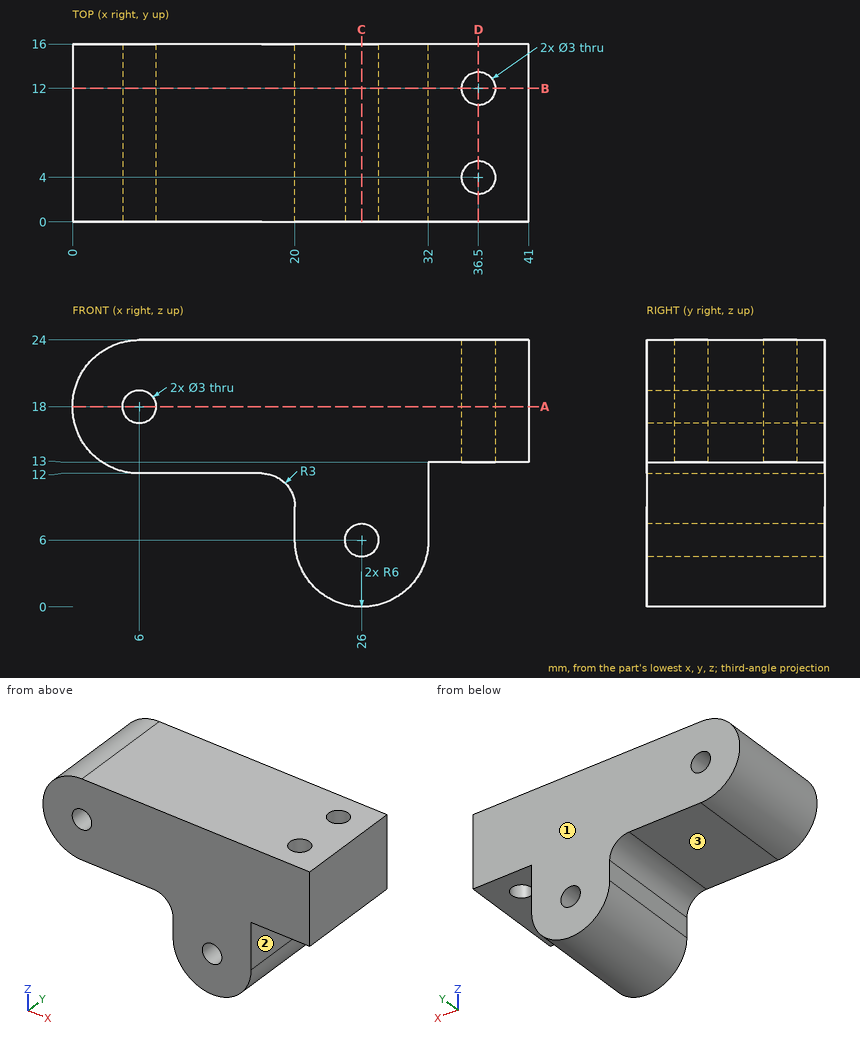
For this review, use the dimensioned drawing (mm, ordinates from the lowest corner) and the shaded views. A direction names the side the tool comes from. Round coordinates to 2 decimals unless told otherwise and drop trailing zeros. Order: outer loops, then holes, each group sorted by start corner. A loop starts at its lowest first (then second) coordinate and runs counter-clockwise, first axis right, second up. Notation, with made-up numbers: (6, -15.75) -> (53, -15.75) arc R29 ccw to (53, 14.25) -> close; hole circle Ø1 at (-20, -38.5). An arc over 180 degrees is marked (long way). One line per item, written item: value. Start each with the question number.
Q1. Take a section at C-C (x = 26). Write out the cut boundary in (y, z).
Q2. Clearance check with flat-ended pins moving along their axes: pin 1 Ø2.5 at (x, z) = (26, 6) entering from -Y; pin 2 Ø5.5 at (y, z) = (6.5, 9.5) entering from +X; pin 3 Ø1.5 at (y, z) = (10.5, 8) entering from -X; pin 4 Ø5.5 at (x, y) = (10, 5.5) entering from -Z. State where each tip first meets the part, or that it passes through.
Q3. Wall thickness on line 1 (Y direction, x = 36.5, z = 20.75); line 2 (X direction, y = 4.75, z = 18); line 3 (X direction, y = 10, z = 6): over which ranges is each line inside the solid? List them lowest first.
Q4. Take a section at D-D (x = 36.5). Write out the cut boundary in (y, z).
Q5. Machinability: for the marked faces 1, 2 and 3, which of the approach directions +Z, -Z, +X, -X, +Y, -Y give a long, thin tool a straight path to every point of the face, cutting with its end or side? Answer none if there is none.
Q6. Take a section at A-A (z = 18). Write out the cut boundary in (x, y), and give its area (3 significant figures).
Q7. Take a section at B-B (y = 12). Write out the cut boundary in (x, z).
Reported:
1. outline: (0, 0) -> (16, 0) -> (16, 4.5) -> (0, 4.5) -> close; (0, 7.5) -> (16, 7.5) -> (16, 24) -> (0, 24) -> close
2. pin 1: passes through
2. pin 2: stops at x = 32
2. pin 3: stops at x = 20
2. pin 4: stops at z = 12
3. line 1: y = 0 to 2.5, 5.5 to 10.5, 13.5 to 16
3. line 2: x = 0 to 4.5, 7.5 to 35.2, 37.8 to 41
3. line 3: x = 20 to 24.5, 27.5 to 32
4. outline: (0, 13) -> (2.5, 13) -> (2.5, 24) -> (0, 24) -> close; (5.5, 13) -> (10.5, 13) -> (10.5, 24) -> (5.5, 24) -> close; (13.5, 13) -> (16, 13) -> (16, 24) -> (13.5, 24) -> close
5. face 1: +Z, -Z, +X, -X, +Y
5. face 2: -Z, +X, +Y, -Y
5. face 3: -Z, -X, +Y, -Y
6. outline: (0, 0) -> (4.5, 0) -> (4.5, 16) -> (0, 16) -> close; (7.5, 0) -> (41, 0) -> (41, 16) -> (7.5, 16) -> close; hole circle Ø3 at (36.5, 4); hole circle Ø3 at (36.5, 12)
6. area: 594 mm2
7. outline: (6, 12) -> (17, 12) arc R3 cw to (20, 9) -> (20, 6) arc R6 ccw to (32, 6) -> (32, 13) -> (35, 13) -> (35, 24) -> (6, 24) arc R6 ccw to start; (38, 13) -> (41, 13) -> (41, 24) -> (38, 24) -> close; hole circle Ø3 at (6, 18); hole circle Ø3 at (26, 6)
